Part model, mm, in its own coordinate system. Face numbers are marked on the shaded views. A direction names the side the tool comes from. Give positions to 0.01 mm unless a question says otherwise; leave off trailing zeros. Loops run counter-clockwise (first coordinate to the right, second up) from the corner with the lowest first, then second, coordinate; pieces in that order, holes last. Notation, with made-up numbers: (-8.75, 7) -> (-0.75, 7) arc R15 cw to (-0.75, 20) -> close; hole circle Ø4 at (54, -19.5). An arc over 180 degrees is marked (long way). Write item = value, one per line.
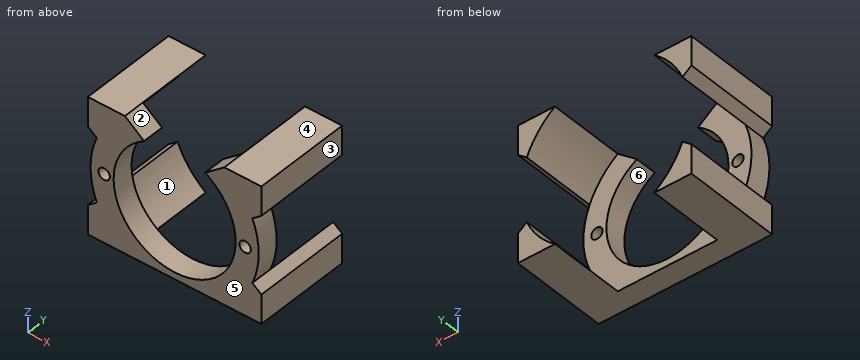
from build123d import *

# Parameters (mm, degrees)
SKETCH1_R           = 2.1
BOSS_EXTRUDE1_DEPTH = 8
BOSS_EXTRUDE2_DEPTH = 36


with BuildPart() as part:
    # Sketch1 → Boss-Extrude1 (new body)
    with BuildSketch(Plane(origin=(0, 0, 0), x_dir=(1, 0, 0), z_dir=(0, 1, 0))):
        with BuildLine():
            Line((18.33030278, -25), (32, -25))
            Line((32, -25), (32, -14.320549047))
            Line((32, -14.320549047), (28.692414075, -11.736497543))
            ThreePointArc((28.692414075, -11.736497543), (31, 0), (28.692414075, 11.736497543))
            Line((28.692414075, 11.736497543), (32, 14.320549047))
            Line((32, 14.320549047), (32, 25))
            Line((32, 25), (-32, 25))
            Line((-32, 25), (-32, 14.320549047))
            Line((-32, 14.320549047), (-28.692414075, 11.736497543))
            ThreePointArc((-28.692414075, 11.736497543), (-31, 0), (-28.692414075, -11.736497543))
            Line((-28.692414075, -11.736497543), (-32, -14.320549047))
            Line((-32, -14.320549047), (-32, -25))
            Line((-32, -25), (-18.33030278, -25))
            Line((-18.33030278, -25), (-11.262551698, -19.478319467))
            ThreePointArc((-11.262551698, -19.478319467), (0, 22.5), (11.262551698, -19.478319467))
            Line((11.262551698, -19.478319467), (18.33030278, -25))
        make_face()
        with Locations(Location((26, 0, 0), (0, 0, 270))):
            Circle(SKETCH1_R, mode=Mode.SUBTRACT)
        with Locations(Location((-26, 0, 0), (0, 0, 270))):
            Circle(SKETCH1_R, mode=Mode.SUBTRACT)
    extrude(amount=BOSS_EXTRUDE1_DEPTH)

    # Sketch1<4> → Boss-Extrude2 (add)
    with BuildSketch(Plane(origin=(0, 0, 0), x_dir=(1, 0, 0), z_dir=(0, 1, 0))):
        with BuildLine():
            Line((28.692414075, 11.736497543), (32, 14.320549047))
            Line((32, 14.320549047), (32, 25))
            Line((32, 25), (18.33030278, 25))
            ThreePointArc((18.33030278, 25), (24.428755585, 19.084965301), (28.692414075, 11.736497543))
        make_face()
        with BuildLine():
            Line((-32, 25), (-32, 14.320549047))
            Line((-32, 14.320549047), (-28.692414075, 11.736497543))
            ThreePointArc((-28.692414075, 11.736497543), (-24.428755585, 19.084965301), (-18.33030278, 25))
            Line((-18.33030278, 25), (-32, 25))
        make_face()
        with BuildLine():
            Line((-32, -14.320549047), (-32, -25))
            Line((-32, -25), (-24.428755585, -19.084965301))
            ThreePointArc((-24.428755585, -19.084965301), (-26.813516388, -15.557484979), (-28.692414075, -11.736497543))
            Line((-28.692414075, -11.736497543), (-32, -14.320549047))
        make_face()
        with BuildLine():
            Line((-32, -25), (-18.33030278, -25))
            ThreePointArc((-18.33030278, -25), (-21.583122502, -22.252389154), (-24.428755585, -19.084965301))
            Line((-24.428755585, -19.084965301), (-32, -25))
        make_face()
        with BuildLine():
            Line((18.33030278, -25), (32, -25))
            Line((32, -25), (32, -14.320549047))
            Line((32, -14.320549047), (28.692414075, -11.736497543))
            ThreePointArc((28.692414075, -11.736497543), (24.428755585, -19.084965301), (18.33030278, -25))
        make_face()
    extrude(amount=BOSS_EXTRUDE2_DEPTH)


solid = part.part
1) Slice it at C-C, the plane x = 26. List the corners of the cut face in (y, z), and give its area (3 significant figures).
Resolved:
outline = (0, -25) -> (36, -25) -> (36, -16.88) -> (8, -16.88) -> (8, -2.1) -> (0, -2.1) -> close; (0, 2.1) -> (8, 2.1) -> (8, 16.88) -> (36, 16.88) -> (36, 25) -> (0, 25) -> close
area = 821 mm²
2) Slice it at B-B, the plane z = 0. List the corners of the cut face in (x, y).
Resolved:
outline = (-31, 0) -> (-28.1, 0) -> (-28.1, 8) -> (-31, 8) -> close; (-23.9, 0) -> (-22.5, 0) -> (-22.5, 8) -> (-23.9, 8) -> close; (22.5, 0) -> (23.9, 0) -> (23.9, 8) -> (22.5, 8) -> close; (28.1, 0) -> (31, 0) -> (31, 8) -> (28.1, 8) -> close
3) Drop flat-ended pins along their axis: P1, Ø2, axis at y = 9, z = -13, coming from the +X side; P2, Ø6.5, axis at x = -26, z = 0, coming from the +Y side; P3, Ø6, axis at x = 8, z = 15.5, coming from the -Y side. Give the stop position or say it passes through.
Resolved:
P1 = 31.59
P2 = 8
P3 = through
4) Pull direction Z, two halves, no side cores. Call the marked faces 4, 5 and 6: pulls with the +Z half, pulls with the -Z half, needs draft (parallel to the pull), parting line crosses it, or undercut.
Resolved:
face_4 = pulls with the +Z half
face_5 = needs draft
face_6 = undercut
5) Which spindle directions (+Z, -Z, +X, -X, +Y, -Y) get a long thin tool onto all of the face, cutting with end or side? Do the marked faces 1, 2 and 3. Say none if no direction does.
Resolved:
face_1 = +Y
face_2 = +Z, +Y, -Y
face_3 = +Z, -Z, +X, +Y, -Y
6) Slice it at D-D, the plane z = -8. List the corners of the cut face in (x, y).
Resolved:
outline = (-29.95, 0) -> (-21.03, 0) -> (-21.03, 8) -> (-29.95, 8) -> close; (21.03, 0) -> (29.95, 0) -> (29.95, 8) -> (21.03, 8) -> close
7) Slice it at A-A, the plane y = 27.5. List the corners of the cut face in (x, z), and give its area (3 significant figures).
Resolved:
outline = (-32, -25) -> (-18.33, -25) arc R31 cw to (-28.69, -11.74) -> (-32, -14.32) -> close; (-32, 14.32) -> (-28.69, 11.74) arc R31 cw to (-18.33, 25) -> (-32, 25) -> close; (18.33, -25) -> (32, -25) -> (32, -14.32) -> (28.69, -11.74) arc R31 cw to start; (18.33, 25) arc R31 cw to (28.69, 11.74) -> (32, 14.32) -> (32, 25) -> close
area = 381 mm²
8) Drill centre lines: line 1 along Z through (x, y) = (0, 4.75); line 2 along Y through (x, z) = (-19, 14.5); line 3 along X through (y, z) = (26, -21.5). Where is each one in solid material? Low to high. Write a range as [from, to].
Resolved:
line_1 = [-25, -22.5]
line_2 = [0, 8]
line_3 = [-32, -22.33], [22.33, 32]
